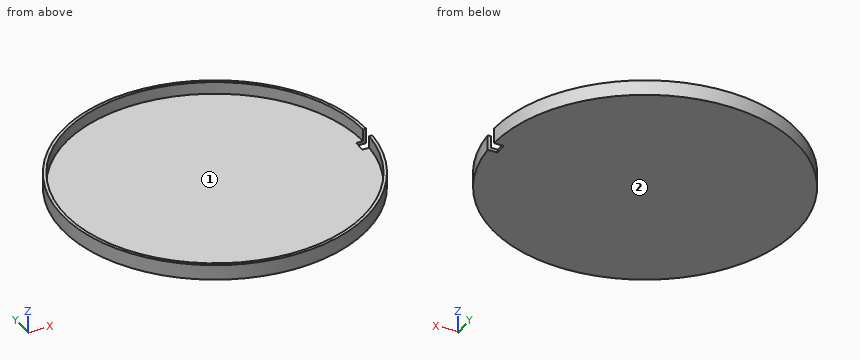
```python
from build123d import *

# Parameters (mm, degrees)
F0_R     = 50
F1_DEPTH = 5
F2_T     = -1
F3_W     = 4
F3_H     = 4
F4_DEPTH = 6


# Not quite as in the source:
# - the program builds the solid bodies; features that only make, move or delete a surface that nothing else refers to are left out


with BuildPart() as f1:
    # F0 (on Top) → F1 (new body)
    with BuildSketch(Plane.XY):
        Circle(F0_R)
    extrude(amount=F1_DEPTH)

    # F2
    f2_openings = [f1.faces().sort_by_distance(p)[0] for p in [
        (0, 0, 5),
    ]]
    offset(amount=F2_T, openings=f2_openings)

    # F3 (on Top) → F4 (cut)
    with BuildSketch(Plane.XY):
        with Locations((48.6989099085, -1.1040147878)):
            Rectangle(F3_W, F3_H)
    extrude(amount=F4_DEPTH, mode=Mode.SUBTRACT)


solid = f1.part
```
CAD build for the part. Positions are in the model's coordinates, mm. Face numbers are marked on the shaded views. Give positions to 0.01 mm unless a question says otherwise; leave off trailing zeros. Order: outer loops, then holes, each group sorted by start corner. A loop starts at its lowest first (then second) coordinate and runs counter-clockwise, first axis right, second up.
(1) Drill centre lines: L1, parallel to Y at x = 0, z = 1.9; L2, parallel to Z at x = -29, y = 17.5; L3, parallel to X at y = 0, z = 2. Where is each one in solid material? Low to high.
(2) Saw through at B-B, the plane y = -40.5. Give the cut face in (x, z).
(3) Saw through at A-A, the plane x = 0. Give the cut face in (y, z).
(4) Flat gauge pins, fed straight in: pin 1 (2 mm diameter, centred on x = -17.5, z = 1, fed in from +Y); pin 2 (3 mm diameter, centred on x = -39.5, y = 21, fed in from +Z); pin 3 (0.8 mm diameter, centred on y = -2, z = 0.5, fed in from +X). Where does each tip first touch, or does it go through?
(5) Mould opens along Y. For the marked faces 1 and 2 say: released by +Y, released by -Y, zero draft, split by the parting line, or undercut.
(6) Saw through at C-C, the plane z = 2.6. Give the cut face in (x, y).
Results found:
1. L1: y = -50 to -49, 49 to 50
1. L2: z = 0 to 1
1. L3: x = -50 to -49
2. outline: (-29.32, 0) - (29.32, 0) - (29.32, 5) - (27.58, 5) - (27.58, 1) - (-27.58, 1) - (-27.58, 5) - (-29.32, 5) - close
3. outline: (-50, 0) - (50, 0) - (50, 5) - (49, 5) - (49, 1) - (-49, 1) - (-49, 5) - (-50, 5) - close
4. pin 1: stops at y = 47.2
4. pin 2: stops at z = 1
4. pin 3: stops at x = 46.7
5. face 1: undercut
5. face 2: zero draft
6. outline: (48.9, -3.1) arc R49 cw (long way) to (48.99, 0.9) - (49.99, 0.9) arc R50 ccw (long way) to (49.9, -3.1) - close
